from build123d import *

# Parameters (mm, degrees)
SKETCH3_W           = 1.15
SKETCH3_H           = 0.25
SKETCH2_OUTSIDE_W   = 29.164
SKETCH2_OUTSIDE_H   = 29.164
SKETCH2_OUTSIDE_W_2 = 13
SKETCH2_OUTSIDE_H_2 = 15
CUT_EXTRUDE1_DEPTH  = 7
CHAMFER1_SIZE       = 0.5


with BuildPart() as part:
    # Sketch1 → Revolve1 (revolve)
    with BuildSketch(Plane.XY):
        Polygon((-18, 0), (-18, 5), (0, 5), (0, 7.5), (9, 7.5), (9, 6), (39, 6), (39, 0), align=None)
    revolve(axis=Axis((-21.980615115, 0, 0), (1, 0, 0)))

    # Sketch3 → Cut-Revolve1 (revolve, cut)
    with BuildSketch(Plane.XY):
        with Locations((35.875, 5.875)):
            Rectangle(SKETCH3_W, SKETCH3_H)
    revolve(axis=Axis((-19.403846942, 0, 0), (1, 0, 0)), mode=Mode.SUBTRACT)

    # Sketch2 outside → Cut-Extrude1 (cut)
    with BuildSketch(Plane(origin=(1, 0, 0), x_dir=(0, 0, -1), z_dir=(1, 0, 0))):
        Rectangle(SKETCH2_OUTSIDE_W, SKETCH2_OUTSIDE_H)
        Rectangle(SKETCH2_OUTSIDE_W_2, SKETCH2_OUTSIDE_H_2, mode=Mode.SUBTRACT)
    extrude(amount=CUT_EXTRUDE1_DEPTH, mode=Mode.SUBTRACT)

    # Chamfer1
    chamfer1_edges = [part.edges().sort_by_distance(p)[0] for p in [
        (39, -6, 0),
        (-18, -5, 0),
    ]]
    chamfer(chamfer1_edges, length=CHAMFER1_SIZE)


solid = part.part
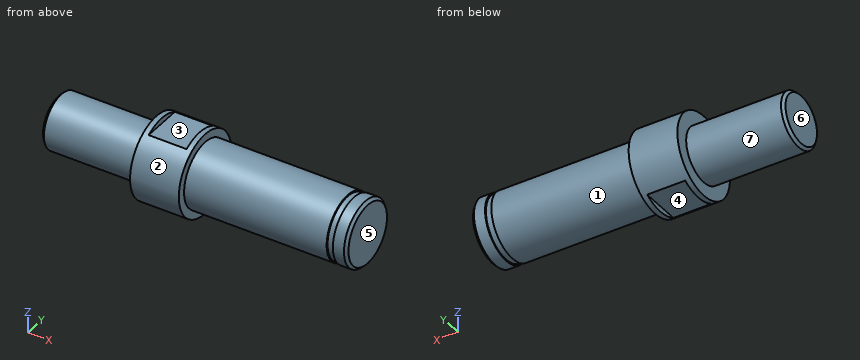
Could you check a few things on this model? Use its own coordinates, in mm. Face numbers are marked on the shaded views. A direction names the side the tool comes from. Give positions to 0.01 mm unless a question says otherwise; leave off trailing zeros. Loops run counter-clockwise (first coordinate to the right, second up) from the corner with the lowest first, then second, coordinate; pieces in that order, holes last. Notation, with made-up numbers: M -3,-22 L 27,-22 A23 ccw 27,5 Z; hole C 62.5,80.5 d3. An arc over 180 degrees is marked long. Answer as a JSON object with one key per item and string values.
Q1. Suppose I cut it at C-C, the plane x = 13. List the corners of the cut face in (y, z) for me, plus the area to 3 significant figures.
Values found:
{"outline": "C 0,0 d12", "area": "113 mm²"}
Q2. If I drill on probe 1 along X at (y, z) = (-2.5, -7); probe 2 along X at (y, z) = (4.75, 1.75); probe 3 along Z at (x, y) = (3.5, -1.75), over which ranges is the centre line in solid material (lowest first)? Write a range as [from, to].
Values found:
{"probe 1": "x = [0, 1], [8, 9]", "probe 2": "x = [0, 39]", "probe 3": "z = [-6.5, 6.5]"}
Q3. If we mould it in two halves opening along X, with no side actions, what happens to the marked faces 4, 5, 6 and 7? For each: pulls with the +X half, pulls with the -X half, needs draft (parallel to the pull), parting line crosses it, or undercut.
Values found:
{"face 4": "undercut", "face 5": "pulls with the +X half", "face 6": "pulls with the -X half", "face 7": "needs draft"}
Q4. Suppose I cut it at D-D, the plane x = 7. List the corners of the cut face in (y, z) for me.
Values found:
{"outline": "M -3.74,-6.5 L 3.74,-6.5 A7.5 ccw 3.74,6.5 L -3.74,6.5 A7.5 ccw Z"}
Q5. For P1, Ø4, axis at x = 5.5, z = 3.5, coming from the +Y side; P2, Ø1.1, axis at y = -1, z = -7, coming from the -X side; P3, Ø3, axis at x = 2, z = 4, coming from the +Y side, each with a flat end and sliding along its axis, tell me the tip position at first contact or that it passes through.
Values found:
{"P1": "stops at y = 7.35", "P2": "stops at x = 0", "P3": "stops at y = 7.07"}
Q6. Suppose I cut it at A-A, the plane z = 0. List the corners of the cut face in (x, y) for me, plus the area to 3 significant figures.
Values found:
{"outline": "M -18,-4.5 L -17.5,-5 L 0,-5 L 0,-7.5 L 9,-7.5 L 9,-6 L 35.3,-6 L 35.3,-5.75 L 36.45,-5.75 L 36.45,-6 L 38.5,-6 L 39,-5.5 L 39,5.5 L 38.5,6 L 36.45,6 L 36.45,5.75 L 35.3,5.75 L 35.3,6 L 9,6 L 9,7.5 L 0,7.5 L 0,5 L -17.5,5 L -18,4.5 Z", "area": "674 mm²"}
Q7. For the marked faces 1, 2 and 3, which set-ups out of +Z, -Z, +X, -X, +Y, -Y let a thin tool reach every point of the face, with its end or its side?
Values found:
{"face 1": "+X", "face 2": "+X, -X", "face 3": "+Z, +Y, -Y"}
